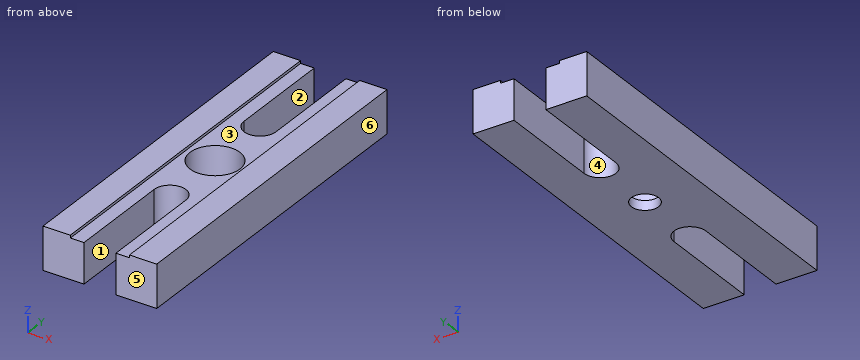
```python
from build123d import *

# Parameters (mm, degrees)
F0_R     = 5.5
F1_DEPTH = 9.4
F0_R_2   = 3
F2_DEPTH = 2.1
F3_R     = 5.5
F4_DEPTH = 0.6


with BuildPart() as f1:
    # F0 (on Top) → F1 (new body)
    with BuildSketch(Plane.XY):
        with BuildLine():
            Line((3.5, -38.1), (12.5, -38.1))
            Line((12.5, -38.1), (12.5, 38.1))
            Line((12.5, 38.1), (3.5, 38.1))
            Line((3.5, 38.1), (3.5, 14.9))
            ThreePointArc((3.5, 14.9), (0, 11.4), (-3.5, 14.9))
            Line((-3.5, 14.9), (-3.5, 38.1))
            Line((-3.5, 38.1), (-12.5, 38.1))
            Line((-12.5, 38.1), (-12.5, -38.1))
            Line((-12.5, -38.1), (-3.5, -38.1))
            Line((-3.5, -38.1), (-3.5, -14.9))
            ThreePointArc((-3.5, -14.9), (0, -11.4), (3.5, -14.9))
            Line((3.5, -14.9), (3.5, -38.1))
        make_face()
        Circle(F0_R, mode=Mode.SUBTRACT)
    extrude(amount=F1_DEPTH)

    # F0 (on Top) → F2 (join)
    with BuildSketch(Plane.XY):
        Circle(F0_R)
        Circle(F0_R_2, mode=Mode.SUBTRACT)
    extrude(amount=F2_DEPTH)

    # F3 (on face) → F4 (cut)
    with BuildSketch(Plane.XY.offset(9.4)):
        with BuildLine():
            Line((6.5, -38.1), (6.5, 38.1))
            Line((6.5, 38.1), (3.5, 38.1))
            Line((3.5, 38.1), (3.5, 14.9))
            ThreePointArc((3.5, 14.9), (0, 11.4), (-3.5, 14.9))
            Line((-3.5, 14.9), (-3.5, 38.1))
            Line((-3.5, 38.1), (-6.5, 38.1))
            Line((-6.5, 38.1), (-6.5, -38.1))
            Line((-6.5, -38.1), (-3.5, -38.1))
            Line((-3.5, -38.1), (-3.5, -14.9))
            ThreePointArc((-3.5, -14.9), (0, -11.4), (3.5, -14.9))
            Line((3.5, -14.9), (3.5, -38.1))
            Line((3.5, -38.1), (6.5, -38.1))
        make_face()
        Circle(F3_R, mode=Mode.SUBTRACT)
    extrude(amount=-F4_DEPTH, mode=Mode.SUBTRACT)


solid = f1.part
```
Check sheet for the modelled part. Datum: model origin and axes. Units: mm. Face numbers are marked on the shaded views. A direction names the side the tool comes from. Round coordinates to 2 decimals unless told otherwise and drop trailing zeros. Loops run counter-clockwise (first coordinate to the right, second up) from the corner with the lowest first, then second, coordinate; pieces in that order, holes last. Notation, with made-up numbers: (10, 49) - (15, 49) arc R24 cw to (15, 81) - close; hole circle Ø3 at (-32.75, 34). An arc over 180 degrees is marked (long way). Answer as a JSON object with one key per item and string values. Group by question number.
Q1. Set-up check for the marked faces 1, 2 and 3: record each of +Z, -Z, +X, -X, +Y, -Y from which the full face is reachable in a straight line by a thin tool's end or side.
Q2. Scan lines: line 1 along X through (y, z) = (-26, 2); line 2 along Y through (x, z) = (-0.25, 8); line 3 along Y through (x, z) = (0, 0.9). Record each from-to range of solid material in increasing order. Write a range as [from, to].
Q3. Mould release check, pull along X, two halves, no side actions. Record for the marked faces 4, 5 and 6: released by +X, released by -X, zero draft, split by the parting line, or undercut.
Q4. Sectioned sample at C-C, the plane z = 1.25. Enter the section's corners in (x, y).
Q5. Sectioned sample at A-A, the plane x = 0. Enter the section's corners in (y, z), plus the area to 3 significant figures.
Q6. Sectioned sample at D-D, the plane y = -20.5. Enter the section's corners in (x, z), plus the area to 3 significant figures.
Q7. Sectioned sample at B-B, the plane y = 0. Enter the section's corners in (x, z), plus the area to 3 significant figures.
Q8. Gauge pin test, flat ends, axial feed: P1, Ø3.5, axis at x = 0, y = 0, coming from the -Z side; P2, Ø1.5, axis at x = 0.5, z = 3.5, coming from the +Y side; P3, Ø9, axis at x = 0, y = 0.5, coming from the +Z side; P4, Ø6.5, axis at x = 2, y = -19, coming from the +Z side. Record the tip position at first contact, or that the pin passes through.
Solution:
{
 "1": {"face 1": "+Z, -Z, -Y", "face 2": "+Z, -Z, +Y", "face 3": "+Z, +Y, -Y"},
 "2": {"line 1": "x = [-12.5, -3.5], [3.5, 12.5]", "line 2": "y = [-11.41, -5.49], [5.49, 11.41]", "line 3": "y = [-11.4, -3], [3, 11.4]"},
 "3": {"face 4": "undercut", "face 5": "zero draft", "face 6": "released by +X"},
 "4": {"outline": "(-12.5, -38.1) - (-3.5, -38.1) - (-3.5, -14.9) arc R3.5 cw to (3.5, -14.9) - (3.5, -38.1) - (12.5, -38.1) - (12.5, 38.1) - (3.5, 38.1) - (3.5, 14.9) arc R3.5 cw to (-3.5, 14.9) - (-3.5, 38.1) - (-12.5, 38.1) - close; hole circle Ø6 at (0, 0)"},
 "5": {"outline": "(-11.4, 0) - (-3, 0) - (-3, 2.1) - (-5.5, 2.1) - (-5.5, 8.8) - (-11.4, 8.8) - close; (3, 0) - (11.4, 0) - (11.4, 8.8) - (5.5, 8.8) - (5.5, 2.1) - (3, 2.1) - close", "area": "114 mm²"},
 "6": {"outline": "(-12.5, 0) - (-3.5, 0) - (-3.5, 8.8) - (-6.5, 8.8) - (-6.5, 9.4) - (-12.5, 9.4) - close; (3.5, 0) - (12.5, 0) - (12.5, 9.4) - (6.5, 9.4) - (6.5, 8.8) - (3.5, 8.8) - close", "area": "166 mm²"},
 "7": {"outline": "(-12.5, 0) - (-3, 0) - (-3, 2.1) - (-5.5, 2.1) - (-5.5, 8.8) - (-6.5, 8.8) - (-6.5, 9.4) - (-12.5, 9.4) - close; (3, 0) - (12.5, 0) - (12.5, 9.4) - (6.5, 9.4) - (6.5, 8.8) - (5.5, 8.8) - (5.5, 2.1) - (3, 2.1) - close", "area": "141 mm²"},
 "8": {"P1": "passes through", "P2": "stops at y = 11.63", "P3": "stops at z = 2.1", "P4": "stops at z = 8.8"}
}
